from build123d import *

# Parameters (mm, degrees)
SKETCH1_R                      = 4.5
BOSSES_DEPTH                   = 5
BOSSES_2_DEPTH                 = 5
BOSSES_3_DEPTH                 = 5
BOSSES_4_DEPTH                 = 5
SKETCH2_W                      = 85
SKETCH2_H                      = 65
BASE_DEPTH                     = 1.2
SKETCH3_R                      = 2.995
INSERT_POCKETS_DEPTH           = 4.7
INSERT_POCKETS_DRAFT           = -2
INSERT_POCKETS_PROFILE_2_DEPTH = 4.7
INSERT_POCKETS_PROFILE_2_DRAFT = -2
INSERT_POCKETS_PROFILE_3_DEPTH = 4.7
INSERT_POCKETS_PROFILE_3_DRAFT = -2
INSERT_POCKETS_PROFILE_4_DEPTH = 4.7
INSERT_POCKETS_PROFILE_4_DRAFT = -2


with BuildPart() as part:
    # Sketch1 → Bosses (new body)
    with BuildSketch(Plane(origin=(0, 0, 0), x_dir=(1, 0, 0), z_dir=(0, 1, 0))):
        with Locations(Location((0, 0, 0), (0, 0, 270))):
            Circle(SKETCH1_R)
    extrude(amount=BOSSES_DEPTH)



with BuildPart() as body_2:
    # Sketch1 → Bosses 2 (new body)
    with BuildSketch(Plane(origin=(0, 0, 0), x_dir=(1, 0, 0), z_dir=(0, 1, 0))):
        with Locations(Location((85, 0, 0), (0, 0, 270))):
            Circle(SKETCH1_R)
    extrude(amount=BOSSES_2_DEPTH)


with BuildPart() as body_3:
    # Sketch1 → Bosses 3 (new body)
    with BuildSketch(Plane(origin=(0, 0, 0), x_dir=(1, 0, 0), z_dir=(0, 1, 0))):
        with Locations(Location((85, 65, 0), (0, 0, 270))):
            Circle(SKETCH1_R)
    extrude(amount=BOSSES_3_DEPTH)


with BuildPart() as body_4:
    # Sketch1 → Bosses 4 (new body)
    with BuildSketch(Plane(origin=(0, 0, 0), x_dir=(1, 0, 0), z_dir=(0, 1, 0))):
        with Locations(Location((0, 65, 0), (0, 0, 270))):
            Circle(SKETCH1_R)
    extrude(amount=BOSSES_4_DEPTH)


with BuildPart() as part_1:
    add(part.part)

    add(body_2.part)  # Base merges body 2

    add(body_3.part)  # Base merges body 3

    add(body_4.part)  # Base merges body 4
    # Sketch2 → Base (add)
    with BuildSketch(Plane(origin=(0, 0, 0), x_dir=(1, 0, 0), z_dir=(0, 1, 0))):
        with Locations((42.5, 32.5)):
            Rectangle(SKETCH2_W, SKETCH2_H)
    extrude(amount=BASE_DEPTH)


with BuildPart() as insert_pockets_tool:
    # Sketch3 → Insert pockets (with draft: the straight prism first)
    with BuildSketch(Plane(origin=(0, 5, 0), x_dir=(1, 0, 0), z_dir=(0, 1, 0))):
        with Locations((0, 65)):
            Circle(SKETCH3_R)
    extrude(amount=-INSERT_POCKETS_DEPTH)
    # Insert pockets: the draft: its side faces are tilted about the plane it starts from
    insert_pockets_sides = [insert_pockets_tool.faces().sort_by_distance(p)[0] for p in [
        (-2.995, 2.65, -65),
    ]]
    draft(insert_pockets_sides, Plane(origin=(0, 5, 0), x_dir=(1, 0, 0), z_dir=(0, 1, 0)), INSERT_POCKETS_DRAFT)


with BuildPart() as part_2:
    add(part_1.part)

    # Insert pockets: cut by insert_pockets_tool
    add(insert_pockets_tool.part, mode=Mode.SUBTRACT)


with BuildPart() as insert_pockets_profile_2_tool:
    # Sketch3 → Insert pockets profile 2 (with draft: the straight prism first)
    with BuildSketch(Plane(origin=(0, 5, 0), x_dir=(1, 0, 0), z_dir=(0, 1, 0))):
        with Locations((85, 65)):
            Circle(SKETCH3_R)
    extrude(amount=-INSERT_POCKETS_PROFILE_2_DEPTH)
    # Insert pockets profile 2: the draft: its side faces are tilted about the plane it starts from
    insert_pockets_profile_2_sides = [insert_pockets_profile_2_tool.faces().sort_by_distance(p)[0] for p in [
        (82.005, 2.65, -65),
    ]]
    draft(insert_pockets_profile_2_sides, Plane(origin=(0, 5, 0), x_dir=(1, 0, 0), z_dir=(0, 1, 0)), INSERT_POCKETS_PROFILE_2_DRAFT)


with BuildPart() as part_3:
    add(part_2.part)

    # Insert pockets profile 2: cut by insert_pockets_profile_2_tool
    add(insert_pockets_profile_2_tool.part, mode=Mode.SUBTRACT)


with BuildPart() as insert_pockets_profile_3_tool:
    # Sketch3 → Insert pockets profile 3 (with draft: the straight prism first)
    with BuildSketch(Plane(origin=(0, 5, 0), x_dir=(1, 0, 0), z_dir=(0, 1, 0))):
        with Locations((85, 0)):
            Circle(SKETCH3_R)
    extrude(amount=-INSERT_POCKETS_PROFILE_3_DEPTH)
    # Insert pockets profile 3: the draft: its side faces are tilted about the plane it starts from
    insert_pockets_profile_3_sides = [insert_pockets_profile_3_tool.faces().sort_by_distance(p)[0] for p in [
        (82.005, 2.65, 0),
    ]]
    draft(insert_pockets_profile_3_sides, Plane(origin=(0, 5, 0), x_dir=(1, 0, 0), z_dir=(0, 1, 0)), INSERT_POCKETS_PROFILE_3_DRAFT)


with BuildPart() as part_4:
    add(part_3.part)

    # Insert pockets profile 3: cut by insert_pockets_profile_3_tool
    add(insert_pockets_profile_3_tool.part, mode=Mode.SUBTRACT)


with BuildPart() as insert_pockets_profile_4_tool:
    # Sketch3 → Insert pockets profile 4 (with draft: the straight prism first)
    with BuildSketch(Plane(origin=(0, 5, 0), x_dir=(1, 0, 0), z_dir=(0, 1, 0))):
        Circle(SKETCH3_R)
    extrude(amount=-INSERT_POCKETS_PROFILE_4_DEPTH)
    # Insert pockets profile 4: the draft: its side faces are tilted about the plane it starts from
    insert_pockets_profile_4_sides = [insert_pockets_profile_4_tool.faces().sort_by_distance(p)[0] for p in [
        (-2.995, 2.65, 0),
    ]]
    draft(insert_pockets_profile_4_sides, Plane(origin=(0, 5, 0), x_dir=(1, 0, 0), z_dir=(0, 1, 0)), INSERT_POCKETS_PROFILE_4_DRAFT)


with BuildPart() as part_5:
    add(part_4.part)

    # Insert pockets profile 4: cut by insert_pockets_profile_4_tool
    add(insert_pockets_profile_4_tool.part, mode=Mode.SUBTRACT)


solid = part_5.part
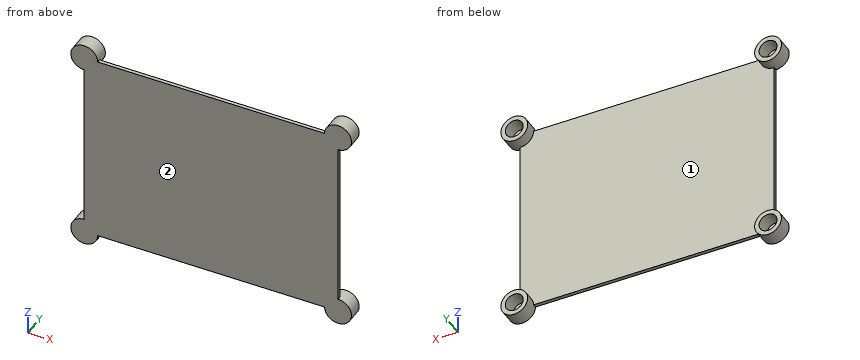
Here's how the part is built. I have some questions about the finished solid (model axes, mm). Face numbers are marked on the shaded views. Coordinates: 2 decimals unless noted, no trailing zeros. Order: outer loops, then holes, each group sorted by start corner. A loop starts at its lowest first (then second) coordinate and runs counter-clockwise, first axis right, second up.
Item 1: If we mould it in two halves opening along Y, with no side actions, what happens to the marked faces 1 and 2? For each: +Y half, -Y half, draft (parallel to the pull), parting line (faces both ways), or undercut.
Result sheet:
face 1: +Y half
face 2: -Y half
Item 2: I need wall thicknesses on line 1 (X direction, y = 1.45, z = -61.5); line 2 (Z direction, x = 22, y = 0.4); line 3 (X direction, y = 0.3, z = -19.5). Which ranges of each line are inside material? Lowest first, please.
Result sheet:
line 1: x = -2.83 to 2.83, 82.17 to 87.83
line 2: z = -65 to 0
line 3: x = 0 to 85
Item 3: If we section it at B-B on z = -40: List the corners of the cut face in (x, y) for me, plus the area to 3 significant figures.
Result sheet:
outline: (0, 0) - (85, 0) - (85, 1.2) - (0, 1.2) - close
area: 102 mm2
Item 4: If we section it at A-A on y = 2.1: List the corners of the cut face in (x, z) for me, plus the area to 3 significant figures.
Result sheet:
outline: circle Ø9 at (0, -65); circle Ø9 at (0, 0); circle Ø9 at (85, -65); circle Ø9 at (85, 0); hole circle Ø5.79 at (0, -65); hole circle Ø5.79 at (0, 0); hole circle Ø5.79 at (85, -65); hole circle Ø5.79 at (85, 0)
area: 149 mm2
Item 5: For P1, Ø3, axis at y = 2, z = -44.5, coming from the +X side; P2, Ø2, axis at x = 70.5, y = 1.5, coming from the -Z side; P3, Ø0.6, axis at x = 46, y = 0.5, coming from the +Z side, each with a flat end and sliding along its axis, tell me the tip position at first contact or that it passes through.
Result sheet:
P1: stops at x = 85
P2: stops at z = -65
P3: stops at z = 0
